Geometry: see drawing. Coordinates: mm, zero at the bounding-box minimum. Round coordinates to 2 decimals unless told otherwise and drop trailing zeros. Order: outer loops, then holes, each group sorted by start corner. A loop starts at its lowest first (then second) coordinate and runs counter-clockwise, first axis right, second up. Notation, with made-up numbers: M 14.25,46.25 L 69.25,46.25 A24 cw 69.25,81.25 Z; hole C 18,69 d2. An arc over 180 degrees is marked long. Answer in a Markdown table with one row per item. Add a question column.
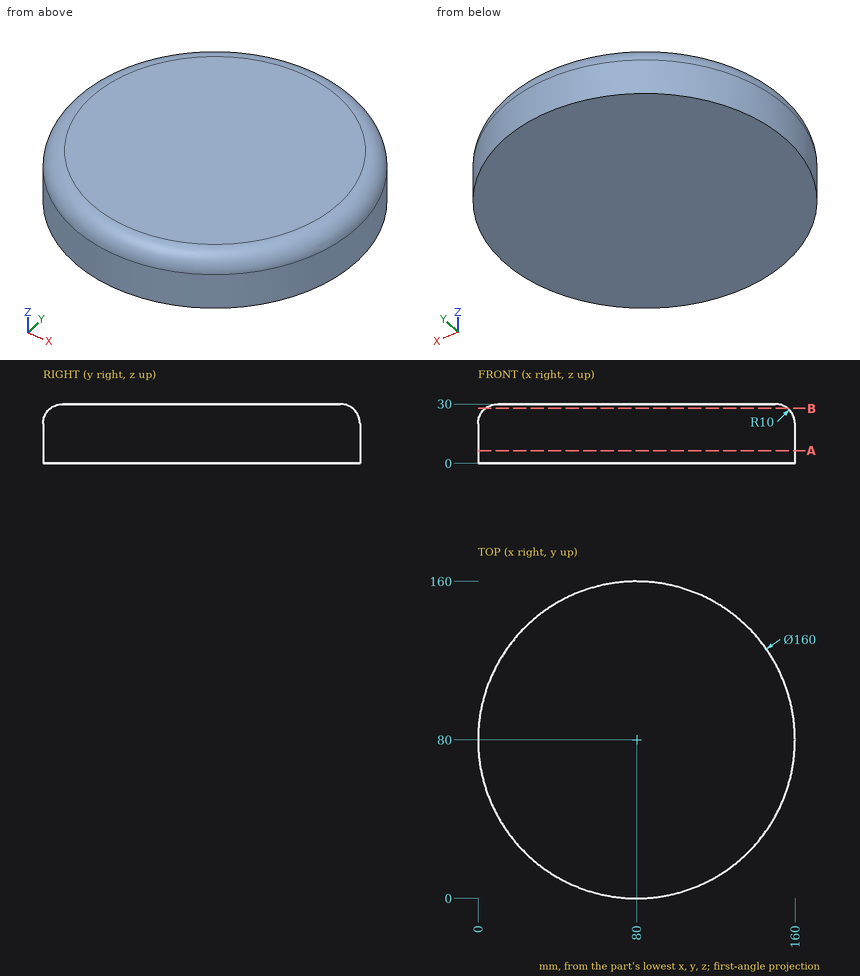
(1) Cut plane B-B (z = 27.75). Return loops of the section in (x, y).
(2) Cut plane A-A (z = 6.5). Return loops of the section in (x, y).
(3) Pin query (flat end, axial travel): pin 1 (10 mm diameter, centred on y = 51, z = 13.5, fed in from +X); pin 2 (12 mm diameter, centred on x = 52.5, z = 18.5, fed in from -Y); pin 3 (3 mm diameter, centred on y = 60, z = 17, fed in from +X). Return the tip coordinate at first contact, or that it passes through.
(4) Line query: line 1 (Y direction, x = 111.5, z = 10); line 2 (X direction, y = 128.5, z = 24); line 3 (X direction, y = 130.5, z = 15.5). Output: solid intervals per line, ascending. Write a range as from..to.
Answer list:
| question | item | result |
|---|---|---|
| 1 | outline | C 80,80 d152.64 |
| 2 | outline | C 80,80 d160 |
| 3 | pin 1 | x = 156.32 |
| 3 | pin 2 | y = 2.94 |
| 3 | pin 3 | x = 157.83 |
| 4 | line 1 | 6.46..153.54 |
| 4 | line 2 | 17.43..142.57 |
| 4 | line 3 | 17.95..142.05 |
